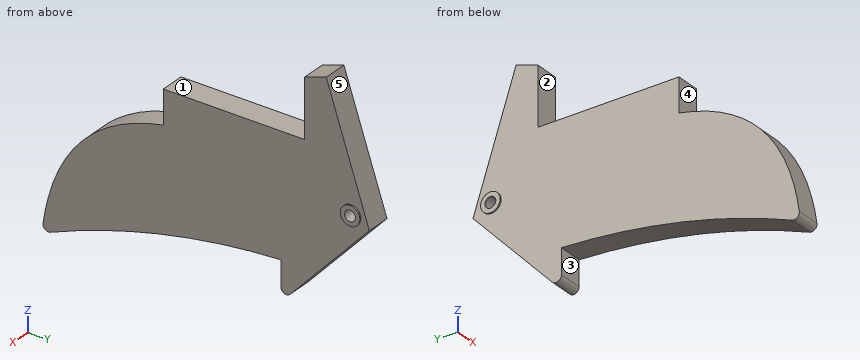
from build123d import *

# Parameters (mm, degrees)
BOSS_EXTRUDE2_DEPTH     = 4.5
SKETCH4_R               = 1
CUT_EXTRUDE2_DEPTH      = 1.0000001
CUT_EXTRUDE2_DEPTH_BACK = 5.5000001
FILLET1_R               = 1
FILLET2_R               = 1
SKETCH5_R               = 1.8
BOSS_EXTRUDE3_DEPTH     = 0.25
SKETCH7_R               = 1
CUT_EXTRUDE3_DEPTH      = 5.7500001


with BuildPart() as part:
    # Sketch3 → Boss-Extrude2 (new body)
    with BuildSketch(Plane(origin=(0, 0, 0), x_dir=(0, 0, -1), z_dir=(1, 0, 0))):
        with BuildLine():
            Line((0, 0), (-23.709832228, -7.927411666))
            Line((-23.709832228, -7.927411666), (-22.370761505, -11.93239381))
            Line((-22.370761505, -11.93239381), (-11.685771853, -11.93239381))
            Line((-11.685771853, -11.93239381), (-11.685771853, -37.874021232))
            Line((-11.685771853, -37.874021232), (-5.488568376, -37.874021232))
            add(Edge.make_bspline(
                [(-5.488568376, -37.874021232), (-1.643222614, -57.890316076), (20.496609615, -60.199338536)],
                knots=[0, 0, 0, 1, 1, 1], degree=2))
            add(Edge.make_bspline(
                [(20.496609615, -60.199338536), (11.480964524, -39.196951523), (10.423170282, -16.267555055)],
                knots=[0, 0, 0, 1, 1, 1], degree=2))
            Line((10.423170282, -16.267555055), (17.625325674, -16.267555055))
            Line((17.625325674, -16.267555055), (0, 0))
        make_face()
    extrude(amount=BOSS_EXTRUDE2_DEPTH)

    # Sketch4 → Cut-Extrude2 (cut, two sides)
    with BuildSketch(Plane(origin=(4.5, 0, 0), x_dir=(0, 0, -1), z_dir=(1, 0, 0))) as cut_extrude2_sk:
        with Locations((-1.549252561, -3.372235527)):
            Circle(SKETCH4_R)
    extrude(amount=CUT_EXTRUDE2_DEPTH, mode=Mode.SUBTRACT)
    extrude(cut_extrude2_sk.sketch, amount=-CUT_EXTRUDE2_DEPTH_BACK, mode=Mode.SUBTRACT)

    # Fillet1
    fillet1_edges = [part.edges().sort_by_distance(p)[0] for p in [
        (2.25, -16.267555055, -17.625325674),
    ]]
    fillet(fillet1_edges, radius=FILLET1_R)

    # Fillet2
    fillet2_edges = [part.edges().sort_by_distance(p)[0] for p in [
        (2.25, -60.199338536, -20.496609615),
    ]]
    fillet(fillet2_edges, radius=FILLET2_R)

    # Sketch5 → Boss-Extrude3 (add)
    with BuildSketch(Plane(origin=(4.5, 0, 0), x_dir=(0, 0, -1), z_dir=(1, 0, 0))):
        with Locations((-1.549252561, -3.372235527)):
            Circle(SKETCH5_R)
    boss_extrude3 = extrude(amount=BOSS_EXTRUDE3_DEPTH)

    # Sketch7 → Cut-Extrude3 (cut, through all)
    with BuildSketch(Plane(origin=(4.75, 0, 0), x_dir=(0, 0, -1), z_dir=(1, 0, 0))):
        with Locations((-1.549252561, -3.372235527)):
            Circle(SKETCH7_R)
    cut_extrude3 = extrude(amount=-CUT_EXTRUDE3_DEPTH, mode=Mode.SUBTRACT)

    # Mirror1: Boss-Extrude3, Cut-Extrude3 across plane
    add(boss_extrude3.mirror(Plane(origin=(2.25, 0, 0), x_dir=(0, 0, 1), z_dir=(1, 0, 0))))
    add(cut_extrude3.mirror(Plane(origin=(2.25, 0, 0), x_dir=(0, 0, 1), z_dir=(1, 0, 0))), mode=Mode.SUBTRACT)


solid = part.part
CAD build for the part. Positions are in the model's coordinates, mm. Face numbers are marked on the shaded views. A direction names the side the tool comes from. Give positions to 0.01 mm unless a question says otherwise; leave off trailing zeros. Order: outer loops, then holes, each group sorted by start corner. A loop starts at its lowest first (then second) coordinate and runs counter-clockwise, first axis right, second up. Notation, with made-up numbers: (56, 78.5) -> (106, 78.5) arc R25 cw to (106, 107.5) -> close; hole circle Ø5 at (-22, -19). An arc over 180 degrees is marked (long way). Return JSON: item names as keys, results as strings.
Q1. Drill centre lines: line 1 (X direction, y = -26, z = 8); line 2 (Z direction, x = 0.25, y = -16); line 3 (Z direction, x = 1.2, y = -55.5). Where is each one in solid material? Low to high.
Working result:
{"line 1": "0 to 4.5", "line 2": "-15.75 to 11.69", "line 3": "-18.59 to -5.68"}
Q2. Saw through at A-A (z = 15.5). Write the cut outline in (x, y).
Working result:
{"outline": "(0, -11.93) -> (4.5, -11.93) -> (4.5, -5.18) -> (0, -5.18) -> close"}
Q3. Mould opens along Y. For the marked faces 1, 2 and 3 say: pulls with the +Y half, pulls with the -Y half, needs draft (parallel to the pull), parting line crosses it, or undercut.
Working result:
{"face 1": "needs draft", "face 2": "pulls with the -Y half", "face 3": "undercut"}
Q4. Which spindle directions (+Z, -Z, +X, -X, +Y, -Y) get a long thin tool onto all of the face, cutting with end or side? Do the marked faces 4 and 5. Say none if no direction does.
Working result:
{"face 4": "+Z, +X, -X, -Y", "face 5": "+Z, +X, -X, +Y"}
Q5. Saw through at B-B (y = -10.5). Write the cut outline in (x, z), then the cut area to 3 significant figures.
Working result:
{"outline": "(0, -11.38) -> (4.5, -11.38) -> (4.5, 22.85) -> (0, 22.85) -> close", "area": "154 mm²"}
Q6. Flat gauge pins, fed straight in: pin 1 (10 mm diameter, centred on y = -47, z = -14, fed in from +X); pin 2 (3 mm diameter, centred on x = 4, z = 14, fed in from +Y); pin 3 (1 mm diameter, centred on x = 1, y = -16, fed in from -Z). Where does each tip first touch, or does it go through?
Working result:
{"pin 1": "x = 4.5", "pin 2": "y = -4.18", "pin 3": "z = -16.04"}
